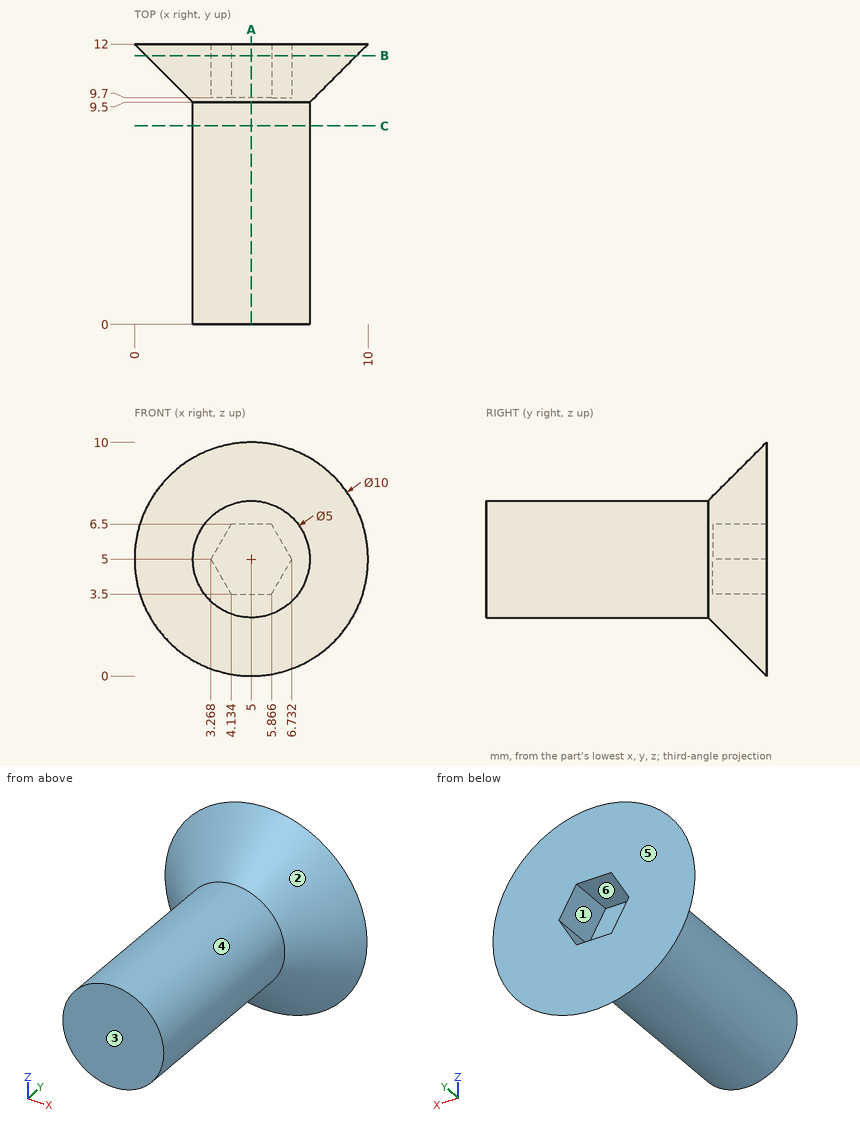
Design review of the part shown in the three views and the two pictorial views. Dimensions are in mm from the part's minimum x, y and z. A direction names the side the tool comes from. Give positions to 0.01 mm unless a question says otherwise; leave off trailing zeros. Write each loop counter-clockwise with the first axis right and the second up, starting at its lowest first coordinate (ties: lowest second). Pieces come first, ordered by that corner, then holes.
Item 1: Wall thickness on probe 1 along Z at (x, y) = (4.5, 10); probe 2 along X at (y, z) = (5, 5); probe 3 along Y at (x, z) = (7.25, 3.5): over which ranges is each line inside the solid? List them lowest first.
Item 2: The part is to be moulded in two halves that separate along X. For the marked faces 1, 2 and 3, say which applies: +X half, -X half, draft (parallel to the pull), parting line (faces both ways), or undercut.
Item 3: Take a section at A-A (x = 5). Give the boundary of the cut face in (y, z).
Item 4: Take a section at C-C (y = 8.5). Give the boundary of the cut face in (x, z), and give its area (3 significant figures).
Item 5: Insertion check: P1, Ø2, axis at x = 5, z = 3, coming from the -Y side; P2, Ø0.9, axis at x = 5, y = 11, coming from the -Z side; P3, Ø0.9, axis at x = 4.5, z = 5.5, coming from the +Y side; P4, Ø2, axis at y = 3.5, z = 6.5, coming from the +X side. Each pin has a flat end and moves straight along its axis. Give the tip position at first contact, or say it passes through.
Item 6: Machinability: for the marked faces 4, 5 and 6, which of the approach directions +Z, -Z, +X, -X, +Y, -Y give a long, thin tool a straight path to every point of the face, cutting with its end or side? Answer none if there is none.
Item 7: Take a section at B-B (y = 11.5). Give the boundary of the cut face in (x, z), and give its area (3 significant figures).
Established:
1. probe 1: z = 2.04 to 3.5, 6.5 to 7.96
1. probe 2: x = 2.5 to 7.5
1. probe 3: y = 9.7 to 12
2. face 1: undercut
2. face 2: parting line
2. face 3: draft
3. outline: (0, 2.5) - (9.5, 2.5) - (12, 0) - (12, 3.5) - (9.7, 3.5) - (9.7, 6.5) - (12, 6.5) - (12, 10) - (9.5, 7.5) - (0, 7.5) - close
4. outline: circle Ø5 at (5, 5)
4. area: 19.6 mm2
5. P1: stops at y = 0
5. P2: stops at z = 0.55
5. P3: stops at y = 9.7
5. P4: stops at x = 7.45
6. face 4: -Y
6. face 5: +Z, -Z, +X, -X, +Y
6. face 6: +Y
7. outline: circle Ø9 at (5, 5); hole (3.27, 5) - (4.13, 3.5) - (5.87, 3.5) - (6.73, 5) - (5.87, 6.5) - (4.13, 6.5) - close
7. area: 55.8 mm2
